from build123d import *

# Parameters (mm, degrees)
SKETCH2_W           = 31.75
SKETCH2_H           = 406.4
BOSS_EXTRUDE1_DEPTH = 25.4
SKETCH3_W           = 25.4
SKETCH3_H           = 22.225
CUT_EXTRUDE1_DEPTH  = 406.4
FILLET1_R           = 2.54
FILLET3_R           = 2.54
SKETCH4_R           = 3.175
CUT_EXTRUDE2_DEPTH  = 50.8


with BuildPart() as part:
    # Sketch2 → Boss-Extrude1 (new body)
    with BuildSketch(Plane(origin=(0, 0, 0), x_dir=(1, 0, 0), z_dir=(0, 1, 0))):
        Rectangle(SKETCH2_W, SKETCH2_H)
    extrude(amount=BOSS_EXTRUDE1_DEPTH)

    # Sketch3 → Cut-Extrude1 (cut)
    with BuildSketch(Plane.XY.offset(203.2)):
        with Locations((0, 14.2875)):
            Rectangle(SKETCH3_W, SKETCH3_H)
    extrude(amount=-CUT_EXTRUDE1_DEPTH, mode=Mode.SUBTRACT)

    # Fillet1
    fillet1_edges = [part.edges().sort_by_distance(p)[0] for p in [
        (-15.875, 0, 0),
        (15.875, 0, 0),
    ]]
    fillet(fillet1_edges, radius=FILLET1_R)

    # Fillet3
    fillet3_edges = [part.edges().sort_by_distance(p)[0] for p in [
        (-12.7, 3.175, 0),
        (12.7, 3.175, 0),
    ]]
    fillet(fillet3_edges, radius=FILLET3_R)

    # Sketch4 → Cut-Extrude2 (cut)
    with BuildSketch(Plane(origin=(15.875, 0, 0), x_dir=(0, 0, -1), z_dir=(1, 0, 0))):
        with Locations((-190.5, 12.7)):
            Circle(SKETCH4_R)
        with Locations((-152.4, 12.7)):
            Circle(SKETCH4_R)
        with Locations((-114.3, 12.7)):
            Circle(SKETCH4_R)
        with Locations((-76.2, 12.7)):
            Circle(SKETCH4_R)
        with Locations((-38.1, 12.7)):
            Circle(SKETCH4_R)
        with Locations((0, 12.7)):
            Circle(SKETCH4_R)
        with Locations((38.1, 12.7)):
            Circle(SKETCH4_R)
        with Locations((76.2, 12.7)):
            Circle(SKETCH4_R)
        with Locations((114.3, 12.7)):
            Circle(SKETCH4_R)
        with Locations((152.4, 12.7)):
            Circle(SKETCH4_R)
        with Locations((190.5, 12.7)):
            Circle(SKETCH4_R)
    extrude(amount=-CUT_EXTRUDE2_DEPTH, mode=Mode.SUBTRACT)


solid = part.part
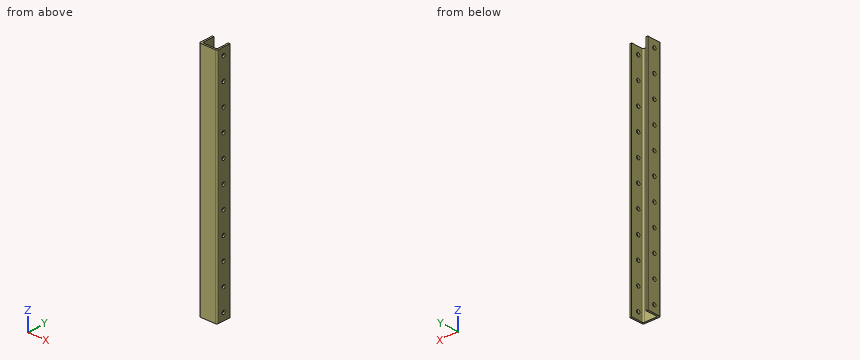
Build history of the part. All positions in model axes, mm. Coordinates: 2 decimals unless noted, no trailing zeros. Write each loop counter-clockwise with the first axis right and the second up, starting at its lowest first coordinate (ties: lowest second). Pieces come first, ordered by that corner, then holes.
(1) Drill centre lines: line 1 (X direction, y = 7.5, z = -83) (3 decimals); line 2 (Y direction, x = -13.4, z = 114.3) (3 decimals); line 3 (Y direction, x = -7, z = 51) (3 decimals). Where is each one in solid material? Low to high.
(2) Cut at B-B on x = 5. List the corners of the cut face in (y, z) (3 decimals).
(3) Pin check, flat tips, straight feed: pin 1 Ø8.5 at (y, z) = (12.7, -76.2) entering from +X (3 decimals); pin 2 Ø6 at (x, z) = (5, -33) entering from +Y (3 decimals). Stop position of each tip, or through.
(4) Cut at A-A on z = 47. List the corners of the cut face in (x, y) (3 decimals).
Working result:
1. line 1: x = -15.875 to -12.7, 12.7 to 15.875
1. line 2: y = 0.001 to 9.525, 15.875 to 25.4
1. line 3: y = 0 to 3.175
2. outline: (0, -203.2) - (3.175, -203.2) - (3.175, 203.2) - (0, 203.2) - close
3. pin 1: stops at x = 15.875
3. pin 2: stops at y = 3.175
4. outline: (-15.875, 2.54) arc R2.54 ccw to (-13.335, 0) - (13.335, 0) arc R2.54 ccw to (15.875, 2.54) - (15.875, 25.4) - (12.7, 25.4) - (12.7, 5.715) arc R2.54 cw to (10.16, 3.175) - (-10.16, 3.175) arc R2.54 cw to (-12.7, 5.715) - (-12.7, 25.4) - (-15.875, 25.4) - close
